Here's how the part is built. I have some questions about the finished solid (model axes, mm). Face numbers are marked on the shaded views. A direction names the side the tool comes from. Coordinates: 2 decimals unless noted, no trailing zeros. Order: outer loops, then holes, each group sorted by start corner. A loop starts at its lowest first (then second) coordinate and runs counter-clockwise, first axis right, second up. Notation, with made-up numbers: (49, -39) - (73, -39) arc R22 ccw to (73, -17) - close; hole circle Ø7 at (31, 41.25). An arc over 180 degrees is marked (long way). Answer in a Markdown table with one row per item. Add a question column.
Item 1: Will these pins go through, and if not, where does the flat tip stop? pin 1 Ø3 at (x, z) = (173.5, -2.5) entering from -Y; pin 2 Ø1 at (y, z) = (132.5, -24.5) entering from -X; pin 3 Ø6.5 at (x, y) = (-27, 252) entering from +Z.
Item 2: I want a section at A-A (y = 22.5). Please give me the cut outline in (x, z) (3 decimals), plus the area to 3 significant figures.
Item 3: On a 3-axis mill with a long thin cutter (end or side, diameter ignored), from which of +Z, -Z, +X, -X, +Y, -Y can I reach the whole of each face in a straight line? I mean the marked faces 1, 2 and 3. Say none if no direction works.
Item 4: If I drill on line 1 along X through (y, z) = (202.5, -112) (3 decimals); line 2 along Z through (x, y) = (135.5, 179), over which ranges is the centre line in solid material (lowest first)? Write a range as from..to.
Item 5: I want a section at C-C (z = -111). Please give me the cut outline in (x, y) (3 decimals).
Item 6: I want a section at D-D (x = 142.5). Please give me the cut outline in (y, z) (3 decimals).
Item 7: I want a section at B-B (z = -37). Please give me the cut outline in (x, y) (3 decimals), plus the area to 3 significant figures.
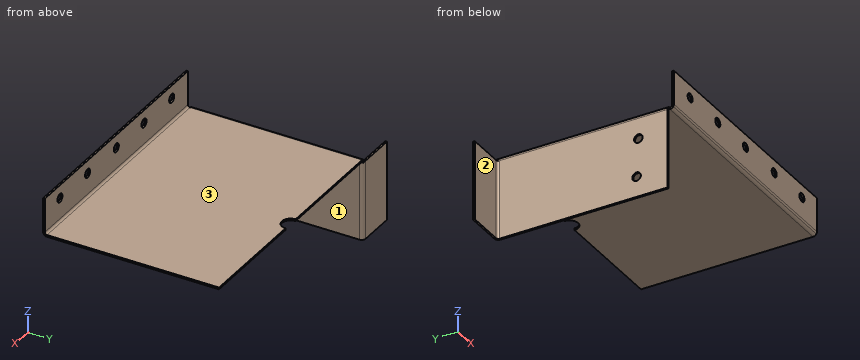
```python
from build123d import *

# Parameters (mm, degrees)
BASE_FLANGE1_DEPTH           = 2.65684
SKETCHED_BEND3_DEPTH         = 360.91368
SKETCHED_BEND3_2_DEPTH       = 360.91368
SKETCH10_R                   = 6.35
CUT_EXTRUDE2_DEPTH           = 2.65684
EDGE_FLANGE5_DEPTH           = 254
EDGE_FLANGE6_STRIP_W         = 16.97736
EDGE_FLANGE6_STRIP_H         = 2.65684
EDGE_FLANGE6_STRIP_CUT_DEPTH = 116.5225
EDGE_FLANGE6_DEPTH           = 116.5225
SKETCH36_R                   = 6.35
CUT_EXTRUDE4_DEPTH           = 2.65684


# Read off the part's stored shape, not the designer's step: Sketched Bend3
# Sheet-metal steps are written as plain solids
with BuildPart() as part:
    # Sketch1 → Base-Flange1 (new body)
    with BuildSketch(Plane.XY):
        with BuildLine():
            Line((0, 0), (0, 254))
            Line((0, 254), (167.75684, 254))
            ThreePointArc((167.75684, 254), (180.45684, 241.3), (193.15684, 254))
            Line((193.15684, 254), (360.91368, 254))
            Line((360.91368, 254), (360.91368, 0))
            Line((360.91368, 0), (360.91368, -57.15))
            Line((360.91368, -57.15), (0, -57.15))
            Line((0, -57.15), (0, 0))
        make_face()
    extrude(amount=-BASE_FLANGE1_DEPTH)

    # Sketched Bend3 outline → Sketched Bend3 (cut)
    with BuildSketch(Plane.YZ):
        with BuildLine():
            ThreePointArc((0, -2.65684), (-2.783367186, -1.949765838), (-4.891802611, 0))
            Line((-4.891802611, 0), (-57.15, 0))
            Line((-57.15, 0), (-57.15, -2.65684))
            Line((-57.15, -2.65684), (0, -2.65684))
        make_face()
    extrude(amount=SKETCHED_BEND3_DEPTH, mode=Mode.SUBTRACT)

    # Sketched Bend3 2 outline → Sketched Bend3 2 (add)
    with BuildSketch(Plane.YZ):
        with BuildLine():
            ThreePointArc((0, 0), (-2.24506403, 0.92993597), (-3.175, 3.175))
            Line((-3.175, 3.175), (-3.175, 53.251044406))
            Line((-3.175, 53.251044406), (-5.83184, 53.251044406))
            Line((-5.83184, 53.251044406), (-5.83184, 3.175))
            ThreePointArc((-5.83184, 3.175), (-5.591894488, 1.519381136), (-4.891802611, 0))
            Line((-4.891802611, 0), (0, 0))
        make_face()
    extrude(amount=SKETCHED_BEND3_2_DEPTH)

    # Sketch10 → Cut-Extrude2 (cut)
    with BuildSketch(Plane(origin=(0, -3.175, 0), x_dir=(1, 0, 0), z_dir=(0, 1, 0))):
        with Locations(Location((322.81368, -34.201044406, 0), (0, 0, 270))):
            Circle(SKETCH10_R)
        with Locations(Location((252.96368, -34.201044406, 0), (0, 0, 270))):
            Circle(SKETCH10_R)
        with Locations(Location((40.75684, -34.201044406, 0), (0, 0, 270))):
            Circle(SKETCH10_R)
        with Locations(Location((110.60684, -34.201044406, 0), (0, 0, 270))):
            Circle(SKETCH10_R)
        with Locations(Location((180.45684, -34.201044406, 0), (0, 0, 270))):
            Circle(SKETCH10_R)
    extrude(amount=-CUT_EXTRUDE2_DEPTH, mode=Mode.SUBTRACT)

    # Edge-Flange5 section (across the edge) → Edge-Flange5 (add)
    with BuildSketch(Plane(origin=(-3.175, 0, -2.65684), x_dir=(1, 0, 0), z_dir=(0, 1, 0))):
        with BuildLine():
            Line((-2.65684, 3.175), (-2.65684, 119.6975))
            Line((-2.65684, 119.6975), (0, 119.6975))
            Line((0, 119.6975), (0, 3.175))
            ThreePointArc((0, 3.175), (0.92993597, 0.92993597), (3.175, 0))
            Line((3.175, 0), (3.175, -2.65684))
            ThreePointArc((3.175, -2.65684), (-0.948733611, -0.948733611), (-2.65684, 3.175))
        make_face()
    extrude(amount=EDGE_FLANGE5_DEPTH)

    # Edge-Flange6 strip (across the edge) → Edge-Flange6 strip cut (cut)
    with BuildSketch(Plane(origin=(-5.83184, 254, -5.83184), x_dir=(0, -1, 0), z_dir=(0, 0, -1))):
        with Locations((-2.65684, -1.32842)):
            Rectangle(EDGE_FLANGE6_STRIP_W, EDGE_FLANGE6_STRIP_H)
    extrude(amount=EDGE_FLANGE6_STRIP_CUT_DEPTH, mode=Mode.SUBTRACT)

    # Edge-Flange6 section (across the edge) → Edge-Flange6 (add)
    with BuildSketch(Plane(origin=(-5.83184, 254, -5.83184), x_dir=(0, -1, 0), z_dir=(0, 0, -1))):
        with BuildLine():
            Line((0, 3.175), (0, 57.15))
            Line((0, 57.15), (2.65684, 57.15))
            Line((2.65684, 57.15), (2.65684, 3.175))
            ThreePointArc((2.65684, 3.175), (3.58677597, 0.92993597), (5.83184, 0))
            Line((5.83184, 0), (5.83184, -2.65684))
            ThreePointArc((5.83184, -2.65684), (1.708106389, -0.948733611), (0, 3.175))
        make_face()
    extrude(amount=EDGE_FLANGE6_DEPTH)

    # Sketch36 → Cut-Extrude4 (cut)
    with BuildSketch(Plane.ZY.offset(5.83184)):
        with Locations((-35.989590501, 43.324159587)):
            Circle(SKETCH36_R)
        with Locations((-92.124928486, 45.966665125)):
            Circle(SKETCH36_R)
    extrude(amount=-CUT_EXTRUDE4_DEPTH, mode=Mode.SUBTRACT)


solid = part.part
```
Values follow:
| question | item | result |
|---|---|---|
| 1 | pin 1 | stops at y = -4.07 |
| 1 | pin 2 | stops at x = -5.83 |
| 1 | pin 3 | stops at z = -5.83 |
| 2 | outline | (-5.832, -122.354) - (-3.175, -122.354) - (-3.175, -5.832) arc R3.175 cw to (0, -2.657) - (360.914, -2.657) - (360.914, 0) - (0, 0) arc R5.832 ccw to (-5.832, -5.832) - close |
| 2 | area | 1,290 mm^2 |
| 3 | face 1 | -Z, +X, +Y, -Y |
| 3 | face 2 | +Z, -Z, -X, -Y |
| 3 | face 3 | +Z, +X, -X, +Y |
| 4 | line 1 | x = -5.832..-3.175 |
| 4 | line 2 | z = -2.66..0 |
| 5 | outline | (-62.982, 251.343) - (-9.007, 251.343) arc R3.175 cw to (-5.832, 248.168) - (-5.832, 0) - (-3.175, 0) - (-3.175, 248.168) arc R5.832 ccw to (-9.007, 254) - (-62.982, 254) - close |
| 6 | outline | (-5.832, 3.175) arc R5.832 ccw to (0, -2.657) - (254, -2.657) - (254, 0) - (0, 0) arc R3.175 cw to (-3.175, 3.175) - (-3.175, 53.251) - (-5.832, 53.251) - close |
| 7 | outline | (-62.982, 251.343) - (-9.007, 251.343) arc R3.175 cw to (-5.832, 248.168) - (-5.832, 49.593) - (-3.175, 49.593) - (-3.175, 248.168) arc R5.832 ccw to (-9.007, 254) - (-62.982, 254) - close; (-5.832, 0) - (-3.175, 0) - (-3.175, 37.055) - (-5.832, 37.055) - close |
| 7 | area | 788 mm^2 |
